```python
from build123d import *

# Parameters (mm, degrees)
CROQUIS1_W              = 73
CROQUIS1_H              = 57.6
SALIENTE_EXTRUIR1_DEPTH = 1.5
CROQUIS3_W              = 73
CROQUIS3_H              = 54.8
SALIENTE_EXTRUIR2_DEPTH = 3
REDONDEO1_R             = 2
REDONDEO4_R             = 0.7
REDONDEO5_R             = 0.7


with BuildPart() as part:
    # Croquis1 → Saliente-Extruir1 (new body)
    with BuildSketch(Plane(origin=(0, 0, 0), x_dir=(1, 0, 0), z_dir=(0, 1, 0))):
        with Locations((36.5, 28.8)):
            Rectangle(CROQUIS1_W, CROQUIS1_H)
    extrude(amount=SALIENTE_EXTRUIR1_DEPTH)

    # Croquis3 → Saliente-Extruir2 (add)
    with BuildSketch(Plane(origin=(0, 0, 0), x_dir=(1, 0, 0), z_dir=(0, 1, 0))):
        with Locations((36.5, 28.9)):
            Rectangle(CROQUIS3_W, CROQUIS3_H)
    extrude(amount=SALIENTE_EXTRUIR2_DEPTH)

    # Redondeo1
    redondeo1_edges = [part.edges().sort_by_distance(p)[0] for p in [
        (73, 3, -28.9),
    ]]
    fillet(redondeo1_edges, radius=REDONDEO1_R)

    # Redondeo4
    redondeo4_edges = [part.edges().sort_by_distance(p)[0] for p in [
        (36.5, 0, 0),
        (36.468245837, 1.5, 0),
    ]]
    fillet(redondeo4_edges, radius=REDONDEO4_R)

    # Redondeo5
    redondeo5_edges = [part.edges().sort_by_distance(p)[0] for p in [
        (36.5, 0, -57.6),
        (36.468245837, 1.5, -57.6),
    ]]
    fillet(redondeo5_edges, radius=REDONDEO5_R)


solid = part.part
```
Work out the finished part from the listing and answer in its coordinate system (mm). A direction names the side the tool comes from. Coordinates: 2 decimals unless noted, no trailing zeros. Loops run counter-clockwise (first coordinate to the right, second up) from the corner with the lowest first, then second, coordinate; pieces in that order, holes last.
1) Flat-ended cylindrical pins translate along their axes: pin 1 (0.9 mm diameter, centred on x = 25, z = -1, fed in from +Y); pin 2 (1.7 mm diameter, centred on x = 21.5, y = 2.5, fed in from -Z); pin 3 (0.5 mm diameter, centred on x = 35.5, z = -56.5, fed in from +Y); pin 4 (1.7 mm diameter, centred on x = 45, y = 2.5, fed in from +Z). Find the tip coordinate at first contact, or state that the pin passes through.
Results:
pin 1: stops at y = 1.5
pin 2: stops at z = -56.3
pin 3: stops at y = 3
pin 4: stops at z = -1.5
2) Consider probe 1 along Z at (x, y) = (5.5, 1.95); probe 2 along X at (y, z) = (1.1, -27.5); probe 3 along X at (y, z) = (1.55, -39.5). Determine where each line is inside the solid, lowest interval first.
Results:
probe 1: z = -56.3 to -1.5
probe 2: x = 0 to 73
probe 3: x = 0 to 72.92
3) Section B-B (y = 2.3) is taken. Give the vertices of the cut face in (x, z), plus the area to 3 significant figures.
Results:
outline: (0, -56.3) - (72.52, -56.3) - (72.52, -1.5) - (0, -1.5) - close
area: 3,970 mm2
4) For faces 1 (the flat face through (36, 2, -56.3)), 2 (the flat face through (36, 2, -1.5)), 3 (the cylindrical face through (72.43, 2.4, -29.2)), determine the directions among +Z, -Z, +X, -X, +Y, -Y from which every point of the face is accessible in a straight line to the end or side of a thin tool.
Results:
face 1: -Z, +X, -X, +Y
face 2: +Z, +X, -X, +Y
face 3: +Z, -Z, +X, +Y
5) Section A-A (x = 66.5) is taken. Give the vertices of the cut face in (y, z), plus the area to 3 significant figures.
Results:
outline: (0, -56.9) arc R0.7 ccw to (0.7, -57.6) - (0.8, -57.6) arc R0.7 ccw to (1.5, -56.9) - (1.5, -56.3) - (3, -56.3) - (3, -1.5) - (1.5, -1.5) - (1.5, -0.7) arc R0.7 ccw to (0.8, 0) - (0.7, 0) arc R0.7 ccw to (0, -0.7) - close
area: 168 mm2
